Verification items for the finished model (mm, model axes). A direction names the side the tool comes from. Round coordinates to 2 decimals unless told otherwise and drop trailing zeros. Write each loop counter-clockwise with the first axis right and the second up, starting at its lowest first coordinate (ties: lowest second). Pieces come first, ordered by that corner, then holes. Notation, with made-up numbers: (23, 8.5) -> (30, 8.5) arc R13 ccw to (30, 21.5) -> close; hole circle Ø4 at (-7.75, 42). An arc over 180 degrees is marked (long way). Answer as a JSON object with one key per item and string values. Group by question number.
(1) Sectioned sample at A-A on x = 61.5. Record the cut outline in (y, z) (3 decimals), and give its area (3 significant figures).
(2) Sectioned sample at D-D on x = 14. Record the cut outline in (y, z) (3 decimals).
(3) Sectioned sample at B-B on x = 89.5. Record the cut outline in (y, z) (3 decimals), and give its area (3 significant figures).
(4) Sectioned sample at C-C on z = 1. Count the separate pieces of the cut face and the enclosed holes in it, and give its area (3 significant figures).
(5) Gauge pin test, flat ends, axial feed: pin 1 Ø0.9 at (y, z) = (29, 1.5) entering from -X; pin 2 Ø2.5 at (x, y) = (51.5, 0) entering from +Z; pin 3 Ø1 at (x, z) = (22, 0.5) entering from +Y (3 decimals); pin 4 Ø1.5 at (x, z) = (18.5, 1) entering from -Y (3 decimals). Record the tip position at first contact, or that the pin passes through.
(6) Scan lines: L1, parallel to X at y = 17, z = 0.1; L2, parallel to X at y = 25, z = 1.25; L3, parallel to X at y = -7, z = 2.45. Record each from-to range of solid material in increasing order. Write a range as from..to.
(7) Draft check along X on faces 3 (the face through (63.81, -0.96, 1.48)), 4 (the face through (2, 8, 3)). Enter one of: released by +X, released by -X, zero draft, split by the parting line, or undercut.
(8) Set-up check for faces 1 (the face through (-48.2, -23.31, 1.48)), 2 (the face through (2, 8, 0)): record each of +Z, -Z, +X, -X, +Y, -Y from which the full face is reachable in a straight line by a thin tool's end or side.
```python
from build123d import *

# Parameters (mm, degrees)
CROQUIS1_R              = 2.5
CROQUIS1_R_2            = 1.5
CROQUIS1_W              = 20
CROQUIS1_H              = 3.5
CROQUIS1_W_2            = 3.5
CROQUIS1_H_2            = 15.2
SALIENTE_EXTRUIR1_DEPTH = 3
CROQUIS2_W              = 10.5
CROQUIS2_H              = 3
SALIENTE_EXTRUIR2_DEPTH = 3
CROQUIS3_R              = 1.5
CORTAR_EXTRUIR1_DEPTH   = 3
CROQUIS4_R              = 1.5
CORTAR_EXTRUIR2_DEPTH   = 3


with BuildPart() as part:
    # Croquis1 → Saliente-Extruir1 (new body)
    with BuildSketch(Plane.XY):
        with BuildLine():
            Line((123, -27.625), (50, -27.625))
            Line((50, -27.625), (50, -27.595))
            ThreePointArc((50, -27.595), (48.242640687, -23.352359313), (44, -21.595))
            Line((44, -21.595), (-44, -21.595))
            ThreePointArc((-44, -21.595), (-48.242640687, -23.352359313), (-50, -27.595))
            Line((-50, -27.595), (-50, -27.625))
            Line((-50, -27.625), (-123, -27.625))
            Line((-123, -27.625), (-123, 27.625))
            Line((-123, 27.625), (-44.2, 27.625))
            Line((-44.2, 27.625), (-44.2, 24.625))
            Line((-44.2, 24.625), (-45.7, 24.625))
            Line((-45.7, 24.625), (-45.7, 21.625))
            Line((-45.7, 21.625), (-39.7, 21.625))
            Line((-39.7, 21.625), (-39.7, 24.625))
            Line((-39.7, 24.625), (-41.2, 24.625))
            Line((-41.2, 24.625), (-41.2, 27.625))
            Line((-41.2, 27.625), (41.2, 27.625))
            Line((41.2, 27.625), (41.2, 24.625))
            Line((41.2, 24.625), (39.7, 24.625))
            Line((39.7, 24.625), (39.7, 21.625))
            Line((39.7, 21.625), (45.7, 21.625))
            Line((45.7, 21.625), (45.7, 24.625))
            Line((45.7, 24.625), (44.2, 24.625))
            Line((44.2, 24.625), (44.2, 27.625))
            Line((44.2, 27.625), (123, 27.625))
            Line((123, 27.625), (123, -27.625))
        make_face()
        with Locations((61.5, 0)):
            Circle(CROQUIS1_R, mode=Mode.SUBTRACT)
        with Locations((71.5, 0)):
            Circle(CROQUIS1_R_2, mode=Mode.SUBTRACT)
        with Locations((51.5, 0)):
            Circle(CROQUIS1_R_2, mode=Mode.SUBTRACT)
        with Locations((-71.5, 0)):
            Circle(CROQUIS1_R_2, mode=Mode.SUBTRACT)
        with Locations((-61.5, 0)):
            Circle(CROQUIS1_R, mode=Mode.SUBTRACT)
        with Locations((-51.5, 0)):
            Circle(CROQUIS1_R_2, mode=Mode.SUBTRACT)
        Polygon((-10, 7.5), (10, 7.5), (10, 4.5), (7.5, 4.5), (7.5, -4.5), (10, -4.5), (10, -7.5), (-10, -7.5), (-10, -4.5), (-7.5, -4.5), (-7.5, 4.5), (-10, 4.5), align=None, mode=Mode.SUBTRACT)
        with Locations((30, -14.845)):
            Rectangle(CROQUIS1_W, CROQUIS1_H, mode=Mode.SUBTRACT)
        with Locations((119.5, 15.225)):
            Rectangle(CROQUIS1_W_2, CROQUIS1_H_2, mode=Mode.SUBTRACT)
        with Locations((119.5, -15.225)):
            Rectangle(CROQUIS1_W_2, CROQUIS1_H_2, mode=Mode.SUBTRACT)
        with Locations((-119.5, 15.225)):
            Rectangle(CROQUIS1_W_2, CROQUIS1_H_2, mode=Mode.SUBTRACT)
        with Locations((-119.5, -15.225)):
            Rectangle(CROQUIS1_W_2, CROQUIS1_H_2, mode=Mode.SUBTRACT)
        with Locations((-30, -14.845)):
            Rectangle(CROQUIS1_W, CROQUIS1_H, mode=Mode.SUBTRACT)
    extrude(amount=SALIENTE_EXTRUIR1_DEPTH)

    # Croquis2 → Saliente-Extruir2 (add)
    with BuildSketch(Plane(origin=(0, 27.625, 0), x_dir=(1, 0, 0), z_dir=(0, 1, 0))):
        with Locations((0, -1.5)):
            Rectangle(CROQUIS2_W, CROQUIS2_H)
        with Locations((80.25, -1.5)):
            Rectangle(CROQUIS2_W, CROQUIS2_H)
        with Locations((-80.25, -1.5)):
            Rectangle(CROQUIS2_W, CROQUIS2_H)
    extrude(amount=SALIENTE_EXTRUIR2_DEPTH)

    # Croquis3 → Cortar-Extruir1 (cut)
    with BuildSketch(Plane.XY.offset(3)):
        with Locations((-120, 0)):
            Circle(CROQUIS3_R)
        with Locations(Location((120, 0, 0), (0, 0, 180))):
            Circle(CROQUIS3_R)
    extrude(amount=-CORTAR_EXTRUIR1_DEPTH, mode=Mode.SUBTRACT)

    # Croquis4 → Cortar-Extruir2 (cut)
    with BuildSketch(Plane.XY.offset(3)):
        with Locations((0, -14.845)):
            Circle(CROQUIS4_R)
    extrude(amount=-CORTAR_EXTRUIR2_DEPTH, mode=Mode.SUBTRACT)


solid = part.part
```
Computed values:
{
 "1": {"outline": "(-27.625, 0) -> (-2.5, 0) -> (-2.5, 3) -> (-27.625, 3) -> close; (2.5, 0) -> (27.625, 0) -> (27.625, 3) -> (2.5, 3) -> close", "area": "151 mm2"},
 "2": {"outline": "(-21.595, 0) -> (27.625, 0) -> (27.625, 3) -> (-21.595, 3) -> close"},
 "3": {"outline": "(-27.625, 0) -> (27.625, 0) -> (27.625, 3) -> (-27.625, 3) -> close", "area": "166 mm2"},
 "4": {"separate pieces": "1", "enclosed holes": "16", "area": "12,300 mm2"},
 "5": {"pin 1": "x = -85.5", "pin 2": "through", "pin 3": "y = 27.625", "pin 4": "y = -21.595"},
 "6": {"L1": "-123..-121.25, -117.75..117.75, 121.25..123", "L2": "-123..-44.2, -41.2..41.2, 44.2..123", "L3": "-123..-10, 10..123"},
 "7": {"face 3": "undercut", "face 4": "zero draft"},
 "8": {"face 1": "+Z, -Z, -Y", "face 2": "-Z, +X, -X, +Y, -Y"}
}
